```python
from build123d import *

# Parameters (mm, degrees)
F0_R          = 30
F0_R_2        = 15
F1_DEPTH      = 16
F1_DEPTH_BACK = 8
F3_DEPTH      = 10
F5_COUNT      = 6


with BuildPart() as f1:
    # F0 (on Top) → F1 (new body, two sides)
    with BuildSketch(Plane.XY) as f1_sk:
        Circle(F0_R)
        Circle(F0_R_2, mode=Mode.SUBTRACT)
    extrude(amount=F1_DEPTH)
    extrude(f1_sk.sketch, amount=-F1_DEPTH_BACK)

    # F2 (on Top) → F3 (join)
    with BuildSketch(Plane.XY):
        with BuildLine():
            Line((15, 25.9807621135), (50, 86.6025403784))
            ThreePointArc((50, 86.6025403784), (25.8819045103, 96.5925826289), (0, 100))
            Line((0, 100), (0, 30))
            ThreePointArc((0, 30), (7.7645713531, 28.9777747887), (15, 25.9807621135))
        make_face()
    extrude(amount=F3_DEPTH)

    # F5: F1 ×6 about axis
    f5_axis = Axis((0, 0, 6.2121879309), (0, 0, -1))


with BuildPart() as f1_1:
    add(f1.part)
    for i in range(1, F5_COUNT):
        add(f1.part.rotate(f5_axis, i * 360 / F5_COUNT))


solid = f1_1.part
```
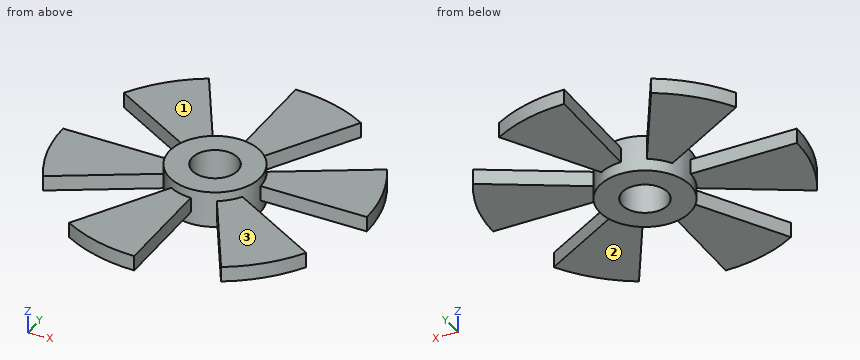
Build history of the part. All positions in model axes, mm. Face numbers are marked on the shaded views. A direction names the side the tool comes from. Give positions to 0.01 mm unless a question says otherwise; leave off trailing zeros. Order: outer loops, then holes, each group sorted by start corner. A loop starts at its lowest first (then second) coordinate and runs counter-clockwise, first axis right, second up. Notation, with made-up numbers: M 56,32 L 102,32 A33 cw 102,70 Z; hole C -12.75,86 d6. An arc over 180 degrees is marked long. Write item = value, one per line. Start each with the question number.
(1) Slice it at C-C on y = 40. Write the cut outline in (x, z).
(2) Probe L1, parallel to Y at x = 0, z = -0.25; L2, parallel to X at y = 39, z = 4; L3, parallel to Y at x = 26, z = 13.25. List the from-to ranges inside material, lowest first. Write a range as [from, to].
(3) Slice it at B-B on y = -7. Write the cut outline in (x, z).
(4) Slice it at A-A on x = -65.5. Write the cut outline in (y, z), plus the area to 3 significant figures.
(5) Pin check, flat tips, straight feed: pin 1 Ø10 at (x, z) = (-6, -3) entering from -Y; pin 2 Ø11 at (x, z) = (-62.5, 4.5) entering from +Y; pin 3 Ø4 at (y, z) = (-26, -5) entering from +X. Stop position of each tip, or through.
(6) Slice it at D-D on z = -5.25. Write the cut outline in (x, y), plus the area to 3 significant figures.
(7) Which spindle directions (+Z, -Z, +X, -X, +Y, -Y) get a long thin tool onto all of the face, cutting with end or side? Do the marked faces 1, 2 and 3. Say none if no direction does.
Responses:
q1.outline = M -69.28,0 L -23.09,0 L -23.09,10 L -69.28,10 Z; M 0,0 L 23.09,0 L 23.09,10 L 0,10 Z; M 69.28,0 L 91.65,0 L 91.65,10 L 69.28,10 Z
q2.L1 = [-30, -15], [15, 30]
q2.L2 = [-67.55, -22.52], [0, 22.52], [67.55, 92.08]
q2.L3 = [-14.97, 14.97]
q3.outline = M -99.75,0 L -29.17,0 L -29.17,-8 L -13.27,-8 L -13.27,16 L -29.17,16 L -29.17,10 L -99.75,10 Z; M 13.27,-8 L 29.17,-8 L 29.17,16 L 13.27,16 Z
q4.outline = M -37.82,0 L 0,0 L 0,10 L -37.82,10 Z; M 37.82,0 L 75.56,0 L 75.56,10 L 37.82,10 Z
q4.area = 756 mm2
q5.pin_1 = -99.98
q5.pin_2 = 82.16
q5.pin_3 = 18
q6.outline = C 0,0 d60; hole C 0,0 d30
q6.area = 2,120 mm2
q7.face_1 = +Z, -X, +Y
q7.face_2 = -Z, +X, -Y
q7.face_3 = +Z, +X, -Y
